Geometry check sheet. Reference: the model listing, model coordinates, mm. A direction names the side the tool comes from. Coordinates: 2 decimals unless noted, no trailing zeros. Loops run counter-clockwise (first coordinate to the right, second up) from the corner with the lowest first, then second, coordinate; pieces in that order, holes last.
from build123d import *

# Parameters (mm, degrees)
SKETCH_W        = 61.15
SKETCH_H        = 54.8
PAD_DEPTH       = 10
POCKET_DEPTH    = 7
SKETCH002_R     = 3.21
SKETCH002_W     = 16.51
SKETCH002_H     = 3.3499967217
POCKET001_DEPTH = 5
SKETCH003_R     = 3.34
SKETCH003_W     = 16.51
SKETCH003_H     = 3.3499967217
POCKET002_DEPTH = 5
SKETCH009_R     = 1.375159
SKETCH009_R_2   = 1.35
PAD003_DEPTH    = 4


with BuildPart() as part:
    # Sketch → Pad (new body)
    with BuildSketch(Plane.XY):
        with Locations((4.8749828339, -3.3899418259)):
            Rectangle(SKETCH_W, SKETCH_H)
    extrude(amount=PAD_DEPTH)

    # Sketch001 (on Face6 of Pad) → Pocket (cut)
    with BuildSketch(Plane.XY.offset(10)):
        with BuildLine():
            ThreePointArc((33.4499828339, 19.4700581741), (32.706036987, 21.2661123273), (30.9099828339, 22.0100581741))
            Line((-21.1600171661, 22.0100581741), (30.9099828339, 22.0100581741))
            ThreePointArc((-21.1600171661, 22.0100581741), (-22.9560771773, 21.2661181853), (-23.7000171661, 19.4700581741))
            Line((-23.7000171661, -26.2499418259), (-23.7000171661, 19.4700581741))
            ThreePointArc((-23.7000171661, -26.2499418259), (-22.9560713193, -28.045995979), (-21.1600171661, -28.7899418259))
            Line((30.2749828339, -28.7899418259), (-21.1600171661, -28.7899418259))
            ThreePointArc((30.2749828339, -28.7899418259), (32.5200439352, -27.8600029272), (33.4499828339, -25.6149418259))
            Line((33.4499828339, 19.4700581741), (33.4499828339, -25.6149418259))
        make_face()
    extrude(amount=-POCKET_DEPTH, mode=Mode.SUBTRACT)

    # Sketch002 (on Face2 of Pocket) → Pocket001 (cut)
    with BuildSketch(Plane(origin=(-25.7000171661, 0, 0), x_dir=(0, -1, 0), z_dir=(-1, 0, 0))):
        with Locations((21.8049418259, 9.1500032783)):
            Circle(SKETCH002_R)
        with Locations((-7.0020581741, 8.3250016391)):
            Rectangle(SKETCH002_W, SKETCH002_H)
    extrude(amount=-POCKET001_DEPTH, mode=Mode.SUBTRACT)

    # Sketch003 (on Face3 of Pocket001) → Pocket002 (cut)
    with BuildSketch(Plane.YZ.offset(35.4499828339)):
        with Locations((-21.8049418259, 10.1500032783)):
            Circle(SKETCH003_R)
        with Locations((-8.7709418259, 9.6500032783)):
            Circle(SKETCH003_R)
        with Locations((6.7920581741, 8.3250016391)):
            Rectangle(SKETCH003_W, SKETCH003_H)
    extrude(amount=-POCKET002_DEPTH, mode=Mode.SUBTRACT)

    # Sketch009 (on Face30 of Pocket002) → Pad003 (join)
    with BuildSketch(Plane.XY.offset(3)):
        with Locations((-7.9520171661, -25.8689418259)):
            Circle(SKETCH009_R)
        with Locations((-7.9520171661, -25.8689418259)):
            Circle(SKETCH009_R_2, mode=Mode.SUBTRACT)
        with Locations((17.5749828339, -25.9959418259)):
            Circle(SKETCH009_R_2)
        with Locations((30.9099828339, 19.4700581741)):
            Circle(SKETCH009_R_2)
        with Locations((-21.1600171661, 19.4700581741)):
            Circle(SKETCH009_R_2)
    extrude(amount=PAD003_DEPTH)


solid = part.part
1) Access from +Z, -Z, +X, -X, +Y, -Y to the whole of each face (thin tool, end or side, straight path). Record for faces 4 (the flat face through (4, -3, 3)), 5 (the flat face through (5, 23, 10)), 6 (the cylindrical face through (-24.71, -21.72, 5.94)).
Data:
face 4: +Z
face 5: +Z, +X, -X, +Y, -Y
face 6: -X
2) Section check A-A on z = 4.25. Record the cut outline in (x, y).
Data:
outline: (-25.7, -30.79) - (35.45, -30.79) - (35.45, 24.01) - (-25.7, 24.01) - close; circle Ø2.7 at (-21.16, 19.47); circle Ø2.75 at (-7.95, -25.87); circle Ø2.7 at (17.57, -26); circle Ø2.7 at (30.91, 19.47); hole (-23.7, -26.25) arc R2.54 ccw to (-21.16, -28.79) - (30.27, -28.79) arc R3.18 ccw to (33.45, -25.61) - (33.45, 19.47) arc R2.54 ccw to (30.91, 22.01) - (-21.16, 22.01) arc R2.54 ccw to (-23.7, 19.47) - close; hole circle Ø2.7 at (-7.95, -25.87)
3) Section check D-D on z = 8. Count the separate pieces of the cut face and the enclosed holes in it, and give its area (3 significant figures).
Data:
separate pieces: 5
enclosed holes: 0
area: 354 mm2
4) Section check C-C on y = -17. Record the cut outline in (x, z), and give its area (3 significant figures).
Data:
outline: (-25.7, 0) - (35.45, 0) - (35.45, 10) - (33.45, 10) - (33.45, 3) - (-23.7, 3) - (-23.7, 10) - (-25.7, 10) - close
area: 211 mm2
5) Mould release check, pull along Y, two halves, no side actions. Record for faces 1 (the flat face through (4, 24.01, 5)), 2 (the flat face through (-25, 15.257, 8)), 3 (the flat face through (35.45, -4, 4)): +Y half, -Y half, draft (parallel to the pull), parting line (faces both ways), or undercut.
Data:
face 1: +Y half
face 2: undercut
face 3: draft
6) Section check B-B on x = -2. Record the cut outline in (y, z).
Data:
outline: (-30.79, 0) - (24.01, 0) - (24.01, 10) - (22.01, 10) - (22.01, 3) - (-28.79, 3) - (-28.79, 10) - (-30.79, 10) - close
7) Depth check by flat-ended pin: pin 1 (2 mm diameter, centred on x = -7.5, y = -25.5, fed in from +Z); pin 2 (4 mm diameter, centred on y = -8.77, z = 9.65, fed in from +X); pin 3 (1 mm diameter, centred on x = 24.5, y = -10, fed in from +Z). Enter the tip coordinate at first touch or a pass-through.
Data:
pin 1: stops at z = 7
pin 2: stops at x = -23.7
pin 3: stops at z = 3
8) Material ranges on probe 1 along X at (y, z) = (-16, 9.25); probe 2 along Y at (x, z) = (-8, 9.25); probe 3 along Z at (x, y) = (-20.5, -14), recorded low to high.
Data:
probe 1: x = -25.7 to -23.7, 33.45 to 35.45
probe 2: y = -30.79 to -28.79, 22.01 to 24.01
probe 3: z = 0 to 3
